from build123d import *

# Parameters (mm, degrees)
SKETCH_1_R      = 1.25
SKETCH_1_R_2    = 1
EXTRUDE_1_DEPTH = 2


with BuildPart() as part:
    # Эскиз1 → Бобышка-Вытянуть1 (new body)
    with BuildSketch(Plane.XY):
        Polygon((15, -49), (15, -28.957842446), (-20.251430991, -28.957842446), (-33.686459833, -42.392871289), (-47.855493079, -49), align=None)
        with Locations((-12.5, -40.578921223)):
            Circle(SKETCH_1_R, mode=Mode.SUBTRACT)
        with Locations((-28.845458385, -44.710050328)):
            Circle(SKETCH_1_R_2, mode=Mode.SUBTRACT)
        with Locations((10.992087761, -34.64156265)):
            Circle(SKETCH_1_R_2, mode=Mode.SUBTRACT)
        Polygon((-10, -36.459984998), (4.798276813, -36.459984998), (4.798276813, -43.678921223), (4.798276813, -44.178921223), (-10, -44.178921223), (-10, -43.678921223), align=None, mode=Mode.SUBTRACT)
    extrude(amount=EXTRUDE_1_DEPTH)


solid = part.part
The model under review builds one solid part; all positions refer to its coordinate system, in mm. A direction names the side the tool comes from. Round coordinates to 2 decimals unless told otherwise and drop trailing zeros. Loops run counter-clockwise (first coordinate to the right, second up) from the corner with the lowest first, then second, coordinate; pieces in that order, holes last. Notation, with made-up numbers: (22, 72) - (75, 72) arc R13 cw to (75, 92) - close; hole circle Ø2 at (6.5, 44). An arc over 180 degrees is marked (long way). Use CSV: the item, a comma, the result in double quotes.
(1) For line 1 (Y direction, x = -7, z = 0.45); line 2 (X direction, y = -40.25, z = 0.7); line 3 (Y direction, x = -12.5, z = 0.8), list the stretches that pass through material, from the lowest coordinate up.
Working result:
line 1,"y = -49 to -44.18, -36.46 to -28.96"
line 2,"x = -31.54 to -13.71, -11.29 to -10, 4.8 to 15"
line 3,"y = -49 to -41.83, -39.33 to -28.96"
(2) The part is to be moulded in two halves that separate along Y. For faces 1 (the flat face through (-40.67, -45.65, 0.99)), 2 (the flat face through (-10, -46, 0)), 3 (the flat face through (4.798, -40, 1)), say which applies: pulls with the +Y half, pulls with the -Y half, needs draft (parallel to the pull), parting line crosses it, or undercut.
Working result:
face 1,"pulls with the +Y half"
face 2,"needs draft"
face 3,"undercut"
(3) Take a section at D-D, the plane y = -31. Give the boundary of the cut face in (x, z), plus the area to 3 significant figures.
Working result:
outline,"(-22.29, 0) - (15, 0) - (15, 2) - (-22.29, 2) - close"
area,"74.6 mm^2"
(4) Clearance check with flat-ended pins moving along their axes: P1, Ø0.6, axis at y = -39.5, z = 0.5, coming from the -X side; P2, Ø12, axis at x = -41.5, y = -36, coming from the -Z side. State where each tip first meets the part, or that it passes through.
Working result:
P1,"stops at x = -31.09"
P2,"passes through"
(5) Take a section at C-C, the plane x = -40. Give the boundary of the cut face in (y, z).
Working result:
outline,"(-49, 0) - (-45.34, 0) - (-45.34, 2) - (-49, 2) - close"
(6) Take a section at B-B, the plane z = 0.85. Give the boundary of the cut face in (x, y), plus the area to 3 significant figures.
Working result:
outline,"(-47.86, -49) - (15, -49) - (15, -28.96) - (-20.25, -28.96) - (-33.69, -42.39) - close; hole circle Ø2 at (-28.85, -44.71); hole circle Ø2.5 at (-12.5, -40.58); hole (-10, -44.18) - (4.8, -44.18) - (4.8, -36.46) - (-10, -36.46) - close; hole circle Ø2 at (10.99, -34.64)"
area,"807 mm^2"
(7) Take a section at A-A, the plane x = -12.5. Give the boundary of the cut face in (y, z), plus the area to 3 significant figures.
Working result:
outline,"(-49, 0) - (-41.83, 0) - (-41.83, 2) - (-49, 2) - close; (-39.33, 0) - (-28.96, 0) - (-28.96, 2) - (-39.33, 2) - close"
area,"35.1 mm^2"
(8) Machinability: for faces 4 (the flat face through (-3, -36.46, 1)), 5 (the flat face through (-10, -46, 2)), which of the approach directions +Z, -Z, +X, -X, +Y, -Y give a long, thin tool a straight path to every point of the face, cutting with its end or side? Answer none if there is none.
Working result:
face 4,"+Z, -Z"
face 5,"+Z, +X, -X, +Y, -Y"
